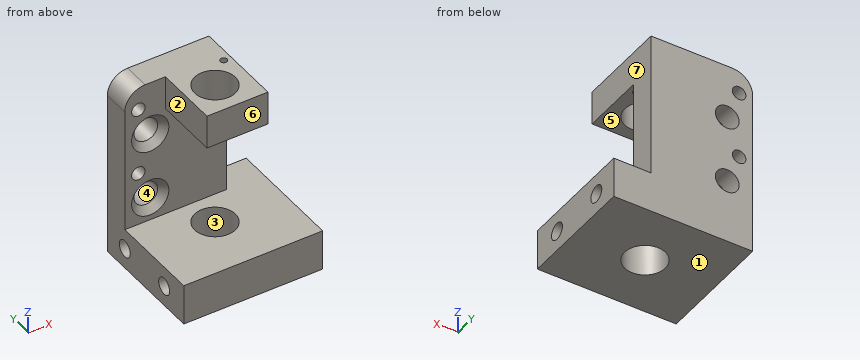
```python
from build123d import *

# Parameters (mm, degrees)
SKETCH_1_W                     = 41
SKETCH_1_H                     = 35
EXTRUDE_1_DEPTH                = 12
SKETCH_2_W                     = 30
SKETCH_2_H                     = 55
EXTRUDE_2_DEPTH                = 8
SKETCH_3_W                     = 18
SKETCH_3_H                     = 19
EXTRUDE_3_DEPTH                = 10
FILLET_1_R                     = 6
F_4_0MM_1_D                    = 4
HOLE_WIZARD_7_0_7_1_AT_2_COUNT = 2
HOLE_WIZARD_7_0_7_1_AT_2_PITCH = 20
SKETCH_9_R                     = 1
CUT_EXTRUDE_1_DEPTH            = 10
HOLE_WIZARD_M6_1_AT_2_COUNT    = 2
HOLE_WIZARD_M6_1_AT_2_PITCH    = 18
SKETCH_12_R                    = 6
CUT_EXTRUDE_2_DEPTH            = 62.249489794


with BuildPart() as part:
    # 草图1 → 凸台-拉伸1 (new body)
    with BuildSketch(Plane.XY):
        Rectangle(SKETCH_1_W, SKETCH_1_H)
    extrude(amount=EXTRUDE_1_DEPTH)

    # 草图2 → 凸台-拉伸2 (add)
    with BuildSketch(Plane(origin=(0, 17.5, 0), x_dir=(1, 0, 0), z_dir=(0, 1, 0))):
        with Locations((-5.5, -27.5)):
            Rectangle(SKETCH_2_W, SKETCH_2_H)
    extrude(amount=-EXTRUDE_2_DEPTH)

    # 草图3 → 凸台-拉伸3 (add)
    with BuildSketch(Plane.XY.offset(55)):
        with Locations((0.5, 0)):
            Rectangle(SKETCH_3_W, SKETCH_3_H)
    extrude(amount=-EXTRUDE_3_DEPTH)

    # 圆角1
    fillet_1_edges = [part.edges().sort_by_distance(p)[0] for p in [
        (-20.5, 13.5, 55),
    ]]
    fillet(fillet_1_edges, radius=FILLET_1_R)

    # Ø4.0mm 暗销孔1 (through all)
    with Locations(Plane(origin=(0, 17.5, 0), x_dir=(1, 0, 0), z_dir=(0, 1, 0))):
        with Locations((-16.5, -48), (-16.5, -28)):
            Hole(F_4_0MM_1_D / 2)

    # 草图8 → Ø7.0 (7) 直径孔1 (revolve, cut)
    with BuildSketch(Plane(origin=(-13, 17.5, 39), x_dir=(0, 0, 1), z_dir=(1, 0, 0))):
        Polygon((0, 0), (0, 8), (5.5, 8), (3.5, 6), (3.5, 0), align=None)
    hole_wizard_7_0_7_1 = revolve(axis=Axis((-13, 23.85, 39), (0, -1, 0)), mode=Mode.SUBTRACT)

    # Ø7.0 (7) 直径孔1 at 2: Ø7.0 (7) 直径孔1 ×2
    with Locations(*[(0, 0, -i * HOLE_WIZARD_7_0_7_1_AT_2_PITCH) for i in range(1, HOLE_WIZARD_7_0_7_1_AT_2_COUNT)]):
        add(hole_wizard_7_0_7_1, mode=Mode.SUBTRACT)

    # 草图9 → 切除-拉伸1 (cut)
    with BuildSketch(Plane.XY.offset(55)):
        with Locations((7.25, 7.25)):
            Circle(SKETCH_9_R)
    extrude(amount=-CUT_EXTRUDE_1_DEPTH, mode=Mode.SUBTRACT)

    # 草图11 → M6 螺纹孔1 (revolve, cut)
    with BuildSketch(Plane(origin=(20.5, 9.5, 6), x_dir=(0, 0, -1), z_dir=(0, 1, 0))):
        Polygon((0, 0), (0, 13.502151548), (2.5, 12), (2.5, 0), align=None)
    hole_wizard_m6_1 = revolve(axis=Axis((26.85, 9.5, 6), (-1, 0, 0)), mode=Mode.SUBTRACT)

    # M6 螺纹孔1 at 2: M6 螺纹孔1 ×2
    with Locations(*[(0, -i * HOLE_WIZARD_M6_1_AT_2_PITCH, 0) for i in range(1, HOLE_WIZARD_M6_1_AT_2_COUNT)]):
        add(hole_wizard_m6_1, mode=Mode.SUBTRACT)

    # 镜向1: M6 螺纹孔1 across plane
    add(hole_wizard_m6_1.mirror(Plane(origin=(0, 0, 0), x_dir=(0, 0, 1), z_dir=(1, 0, 0))), mode=Mode.SUBTRACT)

    # 镜向1 copy 1 sketch → 镜向1 copy 1 (revolve, cut)
    with BuildSketch(Plane(origin=(-20.5, -8.5, 6), x_dir=(0, 0, -1), z_dir=(0, 1, 0))):
        Polygon((0, 0), (0, -13.502151548), (2.5, -12), (2.5, 0), align=None)
    revolve(axis=Axis((-26.85, -8.5, 6), (-1, 0, 0)), mode=Mode.SUBTRACT)

    # 草图12 → 切除-拉伸2 (cut, through all)
    with BuildSketch(Plane.XY.offset(55)):
        Circle(SKETCH_12_R)
    extrude(amount=-CUT_EXTRUDE_2_DEPTH, mode=Mode.SUBTRACT)


solid = part.part
```
Work out the finished part from the listing and answer in its coordinate system (mm). Face numbers are marked on the shaded views. A direction names the side the tool comes from. Round coordinates to 2 decimals unless told otherwise and drop trailing zeros. Loops run counter-clockwise (first coordinate to the right, second up) from the corner with the lowest first, then second, coordinate; pieces in that order, holes last.
(1) For the marked faces 5, 6 and 7, determine the directions among +Z, -Z, +X, -X, +Y, -Y from which every point of the face is accessible in a straight line to the end or side of a thin tool.
Computed values:
face 5: +X, -X, -Y
face 6: +Z, +X, -X, -Y
face 7: +Z, +X, +Y, -Y
(2) Each of these flat-tipped pins is pushed along its axis until it touches: P1, Ø4, axis at y = 9, z = 20, coming from the -X side; P2, Ø12, axis at y = -9.5, z = 44.5, coming from the -X side; P3, Ø4.5, axis at y = -8.5, z = 6, coming from the -X side; P4, Ø4, axis at x = -3.5, z = 34, coming from the -Y side. Where does it stop, or does it pass through?
Computed values:
P1: stops at x = -20.5
P2: stops at x = -8.5
P3: stops at x = -8.35
P4: stops at y = 9.5
(3) The part is cut by section D-D, the plane x = -11. Give the number of separate pieces and of enclosed holes in the cut face, and give its area (3 significant figures).
Computed values:
separate pieces: 3
enclosed holes: 2
area: 624 mm2
(4) Find the intervals of material crossed by L1, parallel to Y at x = -13.25, z = 6; L2, parallel to Z at x = 7, y = 0.5; L3, parallel to Y at x = 0, z = 8.75, in increasing order.
Computed values:
L1: y = -17.5 to -11, -6 to 7, 12 to 17.5
L2: z = 0 to 12, 45 to 55
L3: y = -17.5 to -6, 6 to 17.5
(5) The part is cut by section A-A, the plane y = 0. Give the vertices of the cut face in (x, z).
Computed values:
outline: (-20.5, 0) - (-6, 0) - (-6, 12) - (-20.5, 12) - close; (-8.5, 45) - (-6, 45) - (-6, 55) - (-8.5, 55) - close; (6, 0) - (20.5, 0) - (20.5, 12) - (6, 12) - close; (6, 45) - (9.5, 45) - (9.5, 55) - (6, 55) - close
(6) The part is cut by section B-B, the plane z = 19. Give the vertices of the cut face in (x, y).
Computed values:
outline: (-20.5, 9.5) - (-18.5, 9.5) - (-16.5, 11.5) - (-16.5, 17.5) - (-20.5, 17.5) - close; (-9.5, 11.5) - (-7.5, 9.5) - (9.5, 9.5) - (9.5, 17.5) - (-9.5, 17.5) - close
(7) The part is cut by section C-C, the plane x = 13. Give the vertices of the cut face in (y, z).
Computed values:
outline: (-17.5, 0) - (17.5, 0) - (17.5, 12) - (-17.5, 12) - close; hole circle Ø5 at (-8.5, 6); hole circle Ø5 at (9.5, 6)
(8) The mould has two halves that part along X. Classify the marked faces 1, 2, 3 and 4: pulls with the +X half, pulls with the -X half, needs draft (parallel to the pull), parting line crosses it, or undercut.
Computed values:
face 1: needs draft
face 2: pulls with the -X half
face 3: undercut
face 4: undercut
